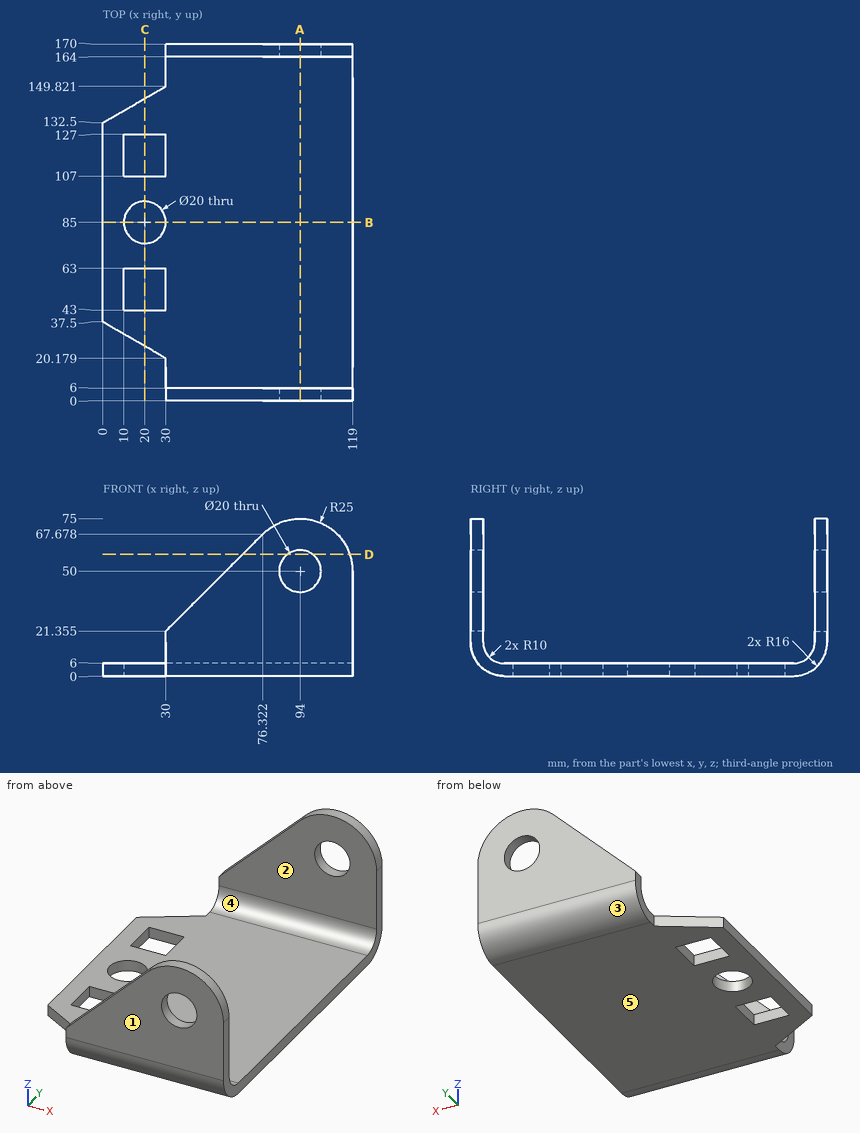
Check sheet for the drawn part. Datum: minimum x, y, z corner. Units: mm. A direction names the side the tool comes from. Coordinates: 2 decimals unless noted, no trailing zeros. Order: outer loops, then holes, each group sorted by start corner. A loop starts at its lowest first (then second) coordinate and runs counter-clockwise, first axis right, second up. Notation, with made-up numbers: (60.5, -29.5) -> (108.5, -29.5) arc R20 ccw to (108.5, -6.5) -> close; hole circle Ø10 at (-26, 72.5). An arc over 180 degrees is marked (long way). Write each question's results on one line, items separated by ' | '. Start each with the question number.
1) Depth check by flat-ended pin: pin 1 (4 mm diameter, centred on x = 28.5, y = 89, fed in from +Z); pin 2 (6 mm diameter, centred on y = 165, z = 15, fed in from -X); pin 3 (5 mm diameter, centred on x = 23.5, z = 3, fed in from +Y); pin 4 (17.5 mm diameter, centred on x = 85.5, z = 58.5, fed in from -Y). Enter the tip coordinate at first touch or a pass-through.
2) Section check B-B (y = 85). Enter the section's corners in (x, z), and give its area (3 significant figures).
3) Section check A-A (x = 94). Enter the section's corners in (y, z).
4) Material ranges on line 1 along Y through (x, z) = (33.5, 20.5); line 2 along Z through (x, y) = (74, 38); line 3 along Z through (x, y) = (94, 1.5) (1 decimal), recorded low to high.
5) Set-up check for the marked faces 4 and 5: record each of +Z, -Z, +X, -X, +Y, -Y from which the full face is reachable in a straight line by a thin tool's end or side.
6) Draft check along Y on the marked faces 1, 2 and 3. Enter one of: pulls with the +Y half, pulls with the -Y half, needs draft (parallel to the pull), parting line crosses it, or undercut.
7) Section check C-C (x = 20). Enter the section's corners in (y, z).
8) Section check D-D (z = 58). Enter the section's corners in (x, y) (1 decimal).
Checked values:
1) pin 1: z = 6 | pin 2: x = 30 | pin 3: y = 147.51 | pin 4: y = 0
2) outline: (0, 0) -> (10, 0) -> (10, 6) -> (0, 6) -> close; (30, 0) -> (119, 0) -> (119, 6) -> (30, 6) -> close | area: 594 mm²
3) outline: (0, 16) arc R16 ccw to (16, 0) -> (154, 0) arc R16 ccw to (170, 16) -> (170, 40) -> (164, 40) -> (164, 16) arc R10 cw to (154, 6) -> (16, 6) arc R10 cw to (6, 16) -> (6, 40) -> (0, 40) -> close; (0, 60) -> (6, 60) -> (6, 75) -> (0, 75) -> close; (164, 60) -> (170, 60) -> (170, 75) -> (164, 75) -> close
4) line 1: 0 to 6, 164 to 170 | line 2: 0 to 6 | line 3: 9.2 to 40, 60 to 75
5) face 4: +Z, +X, -X | face 5: -Z, +X, -X, +Y, -Y
6) face 1: pulls with the -Y half | face 2: undercut | face 3: pulls with the +Y half
7) outline: (25.95, 0) -> (43, 0) -> (43, 6) -> (25.95, 6) -> close; (63, 0) -> (75, 0) -> (75, 6) -> (63, 6) -> close; (95, 0) -> (107, 0) -> (107, 6) -> (95, 6) -> close; (127, 0) -> (144.05, 0) -> (144.05, 6) -> (127, 6) -> close
8) outline: (66.6, 0) -> (88, 0) -> (88, 6) -> (66.6, 6) -> close; (66.6, 164) -> (88, 164) -> (88, 170) -> (66.6, 170) -> close; (100, 0) -> (117.7, 0) -> (117.7, 6) -> (100, 6) -> close; (100, 164) -> (117.7, 164) -> (117.7, 170) -> (100, 170) -> close
